Drawing for the job (mm, zero at the part's lowest x, y, z). Coordinates: 2 decimals unless noted, no trailing zeros. Loops run counter-clockwise (first coordinate to the right, second up) from the corner with the lowest first, then second, coordinate; pieces in that order, holes last. Notation, with made-up numbers: (74, 85) - (101, 85) arc R21 cw to (101, 121) - close; hole circle Ø1 at (-39.75, 41.5). An arc over 180 degrees is marked (long way). One line per item, written item: value.
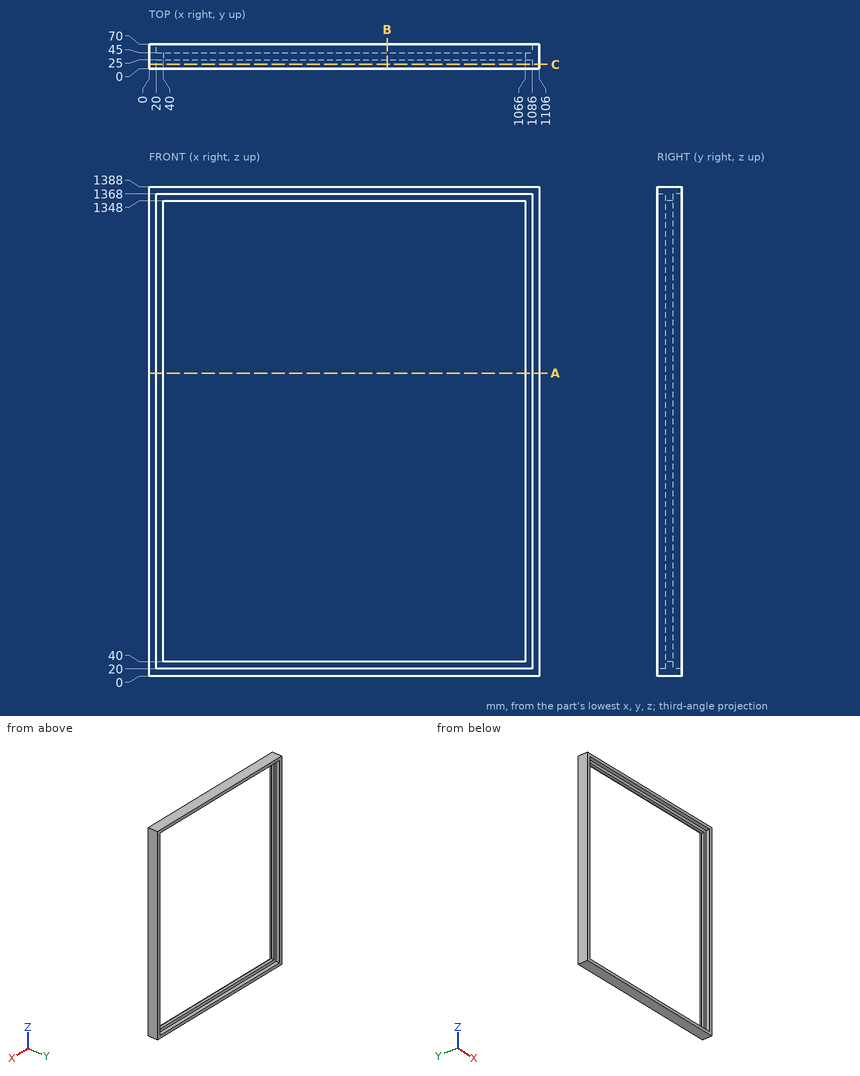
Item 1: Probe probe 1 along X at (y, z) = (4.5, 178.5); probe 2 along X at (y, z) = (41.5, 684); probe 3 along Z at (x, y) = (887.5, 18.5). List the from-to ranges inside material, lowest first. Write a range as from..to.
Check result:
probe 1: x = 0..20, 1086..1106
probe 2: x = 0..40, 1066..1106
probe 3: z = 0..20, 1368..1388
Item 2: Cut at C-C, the plane y = 12. Write the cut outline in (x, z).
Check result:
outline: (0, 0) - (1106, 0) - (1106, 1388) - (0, 1388) - close; hole (20, 20) - (1086, 20) - (1086, 1368) - (20, 1368) - close
Item 3: Cut at A-A, the plane z = 859. Write the cut outline in (x, y), then the cut area to 3 significant figures.
Check result:
outline: (0, 0) - (20, 0) - (20, 25) - (40, 25) - (40, 45) - (20, 45) - (20, 70) - (0, 70) - close; (1066, 25) - (1086, 25) - (1086, 0) - (1106, 0) - (1106, 70) - (1086, 70) - (1086, 45) - (1066, 45) - close
area: 3,600 mm^2
Item 4: Cut at B-B, the plane x = 675. Write the cut outline in (y, z).
Check result:
outline: (0, 0) - (70, 0) - (70, 20) - (45, 20) - (45, 40) - (25, 40) - (25, 20) - (0, 20) - close; (0, 1368) - (25, 1368) - (25, 1348) - (45, 1348) - (45, 1368) - (70, 1368) - (70, 1388) - (0, 1388) - close
Item 5: Drop a flat-ended pin along its axis: P1, Ø6, axis at x = 605.5, y = 36.5, coming from the -Z side. Give the stop position or say it passes through.
Check result:
P1: stops at z = 0
